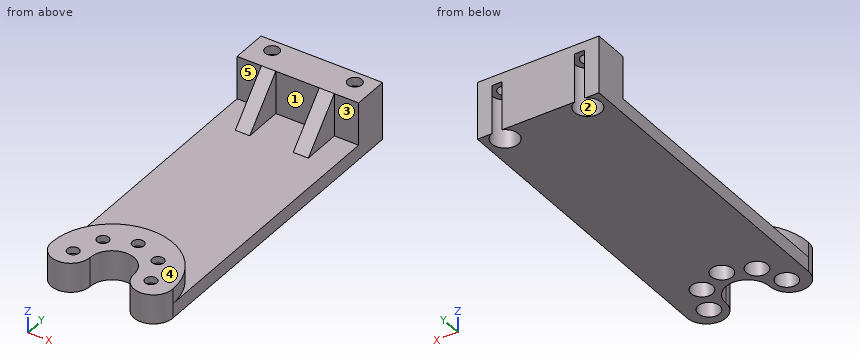
```python
from build123d import *

# Parameters (mm, degrees)
RESSALTO_EXTRUS_O1_DEPTH            = 3.05
RESSALTO_EXTRUS_O2_DEPTH            = 3
ESBO_O4_W                           = 25
ESBO_O4_H                           = 7.35
RESSALTO_EXTRUS_O3_DEPTH            = 11.8
REBAIXO_PARA_SHCS_M2_51_D           = 2.9
REBAIXO_PARA_SHCS_M2_51_CBORE_D     = 5.5
REBAIXO_PARA_SHCS_M2_51_CBORE_DEPTH = 10
REBAIXO_PARA_SHCS_M21_D             = 2.4
REBAIXO_PARA_SHCS_M21_CBORE_D       = 4.4
REBAIXO_PARA_SHCS_M21_CBORE_DEPTH   = 4.7
NERVURA1_REACH                      = 67.869
ESBO_O5_WALL_W                      = 145.630512272
ESBO_O5_WALL_H                      = 15
CORTE_EXTRUS_O1_REACH               = 68.178
ESBO_O6_W                           = 8.93885445
ESBO_O6_H                           = 8


with BuildPart() as part:
    # Esboço1 → Ressalto-extrusão1 (new body)
    with BuildSketch(Plane.XY):
        with BuildLine():
            ThreePointArc((4.5, 0), (0, 4.5), (-4.5, 0))
            ThreePointArc((-4.5, 0), (-8.5, -4), (-12.5, 0))
            ThreePointArc((-12.5, 0), (0, 12.5), (12.5, 0))
            ThreePointArc((12.5, 0), (8.5, -4), (4.5, 0))
        make_face()
    extrude(amount=-RESSALTO_EXTRUS_O1_DEPTH)

    # Esboço2 → Ressalto-extrusão2 (add)
    with BuildSketch(Plane(origin=(0, 0, -3.05), x_dir=(-1, 0, 0), z_dir=(0, 0, -1))):
        with BuildLine():
            Line((-12.5, 64.388275999), (12.5, 64.388275999))
            Line((12.5, 64.388275999), (12.5, 0))
            ThreePointArc((12.5, 0), (8.5, -4), (4.5, 0))
            ThreePointArc((4.5, 0), (0, 4.5), (-4.5, 0))
            ThreePointArc((-4.5, 0), (-8.5, -4), (-12.5, 0))
            Line((-12.5, 0), (-12.5, 64.388275999))
        make_face()
    extrude(amount=RESSALTO_EXTRUS_O2_DEPTH)

    # Esboço4 → Ressalto-extrusão3 (add)
    with BuildSketch(Plane(origin=(0, 0, -6.05), x_dir=(-1, 0, 0), z_dir=(0, 0, -1))):
        with Locations((0, 60.713275999)):
            Rectangle(ESBO_O4_W, ESBO_O4_H)
    extrude(amount=-RESSALTO_EXTRUS_O3_DEPTH)

    # Rebaixo para SHCS M2.51 (through all)
    with Locations(Plane(origin=(0, 0, -6.05), x_dir=(-1, 0, 0), z_dir=(0, 0, -1))):
        with Locations((-8.5, 61.838275999), (8.5, 61.838275999)):
            CounterBoreHole(REBAIXO_PARA_SHCS_M2_51_D / 2, REBAIXO_PARA_SHCS_M2_51_CBORE_D / 2, REBAIXO_PARA_SHCS_M2_51_CBORE_DEPTH)

    # Rebaixo para SHCS M21 (through all)
    with Locations(Plane(origin=(0, 0, -6.05), x_dir=(-1, 0, 0), z_dir=(0, 0, -1))):
        with Locations((-8, 0), (-5.656854249, 5.656854249), (0, 8), (5.656854249, 5.656854249), (8, 0)):
            CounterBoreHole(REBAIXO_PARA_SHCS_M21_D / 2, REBAIXO_PARA_SHCS_M21_CBORE_D / 2, REBAIXO_PARA_SHCS_M21_CBORE_DEPTH)

    # Esboço5 wall → Nervura1 (add, up to next)
    with BuildSketch(Plane(origin=(0, 53.038275999, 1.35), x_dir=(0, -0.672672793996, -0.739940073396), z_dir=(0, 0.739940073396, -0.672672793996)), mode=Mode.PRIVATE) as nervura1_sk1:
        Rectangle(ESBO_O5_WALL_W, ESBO_O5_WALL_H)
    nervura1_tool1 = extrude(nervura1_sk1.sketch, amount=NERVURA1_REACH, mode=Mode.PRIVATE) - part.part
    add(nervura1_tool1.solids().sort_by_distance((0, 53.038275999, 1.35))[0])

    # Esboço6 → Corte-extrusão1 (cut, up to next)
    with BuildSketch(Plane.XY.offset(-3.05), mode=Mode.PRIVATE) as corte_extrus_o1_sk1:
        with Locations((-0.067802218, 53.038275999)):
            Rectangle(ESBO_O6_W, ESBO_O6_H)
    corte_extrus_o1_tool1 = extrude(corte_extrus_o1_sk1.sketch, amount=CORTE_EXTRUS_O1_REACH, mode=Mode.PRIVATE) & part.part
    add(corte_extrus_o1_tool1.solids().sort_by_distance((-0.067802, 53.038276, -3.05))[0], mode=Mode.SUBTRACT)


solid = part.part
```
Work out the finished part from the listing and answer in its coordinate system (mm). Face numbers are marked on the shaded views. A direction names the side the tool comes from. Round coordinates to 2 decimals unless told otherwise and drop trailing zeros. Order: outer loops, then holes, each group sorted by start corner. A loop starts at its lowest first (then second) coordinate and runs counter-clockwise, first axis right, second up.
Q1. A tool of negligible diameter and unlimited length cuts with its end or side. For the marked faces 1, 2, 3, 4 and 5, from which of +Z, -Z, +X, -X, +Y, -Y can it reach the whole face along a straight path? Write none if from no direction.
Solution:
face 1: +Z
face 2: -Z
face 3: +Z, +X
face 4: +Z, +X, -X, -Y
face 5: +Z, -X
Q2. Find the intervals of material crossed by line 1 along Y through (x, z) = (-8.5, 5.35); line 2 along Z through (x, y) = (-10.5, 13); line 3 along Y through (x, z) = (-10, -2.25), in increasing order.
Solution:
line 1: y = 57.04 to 60.39, 63.29 to 64.39
line 2: z = -6.05 to -3.05
line 3: y = -3.71 to -0.92, 0.92 to 7.5, 57.04 to 59.53, 64.14 to 64.39
Q3. Given pin 1 Ø2.5 at (x, y) = (0, 8) entering from -Z; pin 2 Ø1.4 at (x, y) = (-8, 0) entering from +Z; pin 3 Ø7 at (x, y) = (-5.66, 5.66) entering from +Z; pin 4 Ø4 at (y, z) = (54, 0.5) entering from -X, each flat-ended and moving along its own axis, determine where each tip first touches the part or whether it passes through.
Solution:
pin 1: stops at z = -1.35
pin 2: passes through
pin 3: stops at z = 0
pin 4: stops at x = -7.5
Q4. A cutting plane is placed at C-C, the plane z = -4.25. Determine the outline of the cut face in (x, y).
Solution:
outline: (-12.5, 0) arc R4 ccw to (-4.5, 0) arc R4.5 cw to (4.5, 0) arc R4 ccw to (12.5, 0) - (12.5, 64.39) - (9.53, 64.39) arc R2.75 cw (long way) to (7.47, 64.39) - (-7.47, 64.39) arc R2.75 cw (long way) to (-9.53, 64.39) - (-12.5, 64.39) - close; hole circle Ø4.4 at (-8, 0); hole circle Ø4.4 at (-5.66, 5.66); hole circle Ø4.4 at (0, 8); hole circle Ø4.4 at (5.66, 5.66); hole circle Ø4.4 at (8, 0)
Q5. A cutting plane is placed at A-A, the plane x = -8.5. Determine the outline of the cut face in (y, z).
Solution:
outline: (-4, -6.05) - (-2.14, -6.05) - (-2.14, -1.35) - (-1.09, -1.35) - (-1.09, 0) - (-4, 0) - close; (1.09, -1.35) - (2.14, -1.35) - (2.14, -6.05) - (59.09, -6.05) - (59.09, 3.95) - (60.39, 3.95) - (60.39, 5.75) - (57.04, 5.75) - (57.04, -3.05) - (9.17, -3.05) - (9.17, 0) - (1.09, 0) - close; (63.29, 3.95) - (64.39, 3.95) - (64.39, 5.75) - (63.29, 5.75) - close
Q6. A cutting plane is placed at D-D, the plane y = 53. Determine the outline of the cut face in (x, z).
Solution:
outline: (-12.5, -6.05) - (12.5, -6.05) - (12.5, -3.05) - (7.5, -3.05) - (7.5, 1.31) - (4.4, 1.31) - (4.4, -3.05) - (-4.54, -3.05) - (-4.54, 1.31) - (-7.5, 1.31) - (-7.5, -3.05) - (-12.5, -3.05) - close
Q7. A cutting plane is placed at B-B, the plane y = 23. Determine the outline of the cut face in (x, z), then the cut area to 3 significant figures.
Solution:
outline: (-12.5, -6.05) - (12.5, -6.05) - (12.5, -3.05) - (-12.5, -3.05) - close
area: 75.0 mm2
